```python
from build123d import *

# Parameters (mm, degrees)
BOSS_EXTRUDE1_DEPTH  = 6.35
SKETCH2_R            = 17
CUT_EXTRUDE1_DEPTH   = 109.352768769
M5_CLEARANCE_HOLE1_D = 5.5
M5_CLEARANCE_HOLE2_D = 5.5
FILLET1_R            = 5.08


with BuildPart() as part:
    # Sketch1 → Boss-Extrude1 (new body)
    with BuildSketch(Plane(origin=(0, 0, 0), x_dir=(1, 0, 0), z_dir=(0, 1, 0))):
        with BuildLine():
            Line((0, 60), (0, 0))
            Line((0, 0), (60, 0))
            Line((60, 0), (60, 60))
            ThreePointArc((60, 60), (30, 90), (0, 60))
        make_face()
    extrude(amount=BOSS_EXTRUDE1_DEPTH)

    # Sketch2 → Cut-Extrude1 (cut, through all)
    with BuildSketch(Plane(origin=(0, 6.35, 0), x_dir=(1, 0, 0), z_dir=(0, 1, 0))):
        with Locations(Location((30, 60, 0), (0, 0, 270))):
            Circle(SKETCH2_R)
    extrude(amount=-CUT_EXTRUDE1_DEPTH, mode=Mode.SUBTRACT)

    # M5 Clearance Hole1 (through all)
    with Locations(Plane(origin=(0, 6.35, 0), x_dir=(-1, 0, 0), z_dir=(0, 1, 0))):
        with Locations((-15.857864376, -74.142135624), (-44.142135624, -45.857864376), (-44.142135624, -74.142135624), (-15.857864376, -45.857864376), (-30, -80), (-50, -60), (-30, -40), (-10, -60)):
            Hole(M5_CLEARANCE_HOLE1_D / 2)

    # M5 Clearance Hole2 (through all)
    with Locations(Plane(origin=(0, 6.35, 0), x_dir=(-1, 0, 0), z_dir=(0, 1, 0))):
        with Locations((-10.95, -12.7), (-49.05, -12.7)):
            Hole(M5_CLEARANCE_HOLE2_D / 2)

    # Fillet1
    fillet1_edges = [part.edges().sort_by_distance(p)[0] for p in [
        (60, 3.175, 0),
        (0, 3.175, 0),
    ]]
    fillet(fillet1_edges, radius=FILLET1_R)


solid = part.part
```
Geometry: final body of the model. Coordinates: model frame, mm. Round coordinates to 2 decimals unless told otherwise and drop trailing zeros. Order: outer loops, then holes, each group sorted by start corner. A loop starts at its lowest first (then second) coordinate and runs counter-clockwise, first axis right, second up. Notation, with made-up numbers: (34, 79.5) - (72, 79.5) arc R26 ccw to (72, 108.5) - close; hole circle Ø11 at (-11, 12). An arc over 180 degrees is marked (long way). Write item = value, one per line. Start each with the question number.
Q1. Cut plane B-B on z = -12.7. Return the cut outline in (x, y), and give its area (3 significant figures).
Q2. Cut plane D-D on z = -44. Return the cut outline in (x, y).
Q3. Cut plane A-A on x = 30. Return the cut outline in (y, z), and give its area (3 significant figures).
Q4. Ray query, line 1 (X direction, y = 5.25, z = -12.5); line 2 (Z direction, x = 31.5, y = 4); line 3 (Z direction, x = 49.05, y = 3.75). Return the intervals inside material, ascending. Write a range as from..to.
Q5. Cut plane C-C on x = 49.05. Return the cut outline in (y, z).
Q6. Pull-direction query (X, two-part tool) for faces 1 (the cylindrical face through (30.66, 3.131, -89.993)), 2 (the flat face through (60, 3, -32)), 3 (the cylindrical face through (15, 3, -52)); classes: +X half, -X half, draft (parallel to the pull), parting line (faces both ways), or undercut.
Outcome:
q1.outline = (0, 0) - (8.2, 0) - (8.2, 6.35) - (0, 6.35) - close; (13.7, 0) - (46.3, 0) - (46.3, 6.35) - (13.7, 6.35) - close; (51.8, 0) - (60, 0) - (60, 6.35) - (51.8, 6.35) - close
q1.area = 311 mm^2
q2.outline = (0, 0) - (13.83, 0) - (13.83, 6.35) - (0, 6.35) - close; (17.89, 0) - (24.26, 0) - (24.26, 6.35) - (17.89, 6.35) - close; (35.74, 0) - (42.11, 0) - (42.11, 6.35) - (35.74, 6.35) - close; (46.17, 0) - (60, 0) - (60, 6.35) - (46.17, 6.35) - close
q3.outline = (0, -90) - (6.35, -90) - (6.35, -82.75) - (0, -82.75) - close; (0, -77.25) - (6.35, -77.25) - (6.35, -77) - (0, -77) - close; (0, -43) - (6.35, -43) - (6.35, -42.75) - (0, -42.75) - close; (0, -37.25) - (6.35, -37.25) - (6.35, 0) - (0, 0) - close
q3.area = 286 mm^2
q4.line_1 = 0..8.21, 13.69..46.31, 51.79..60
q4.line_2 = -89.96..-82.3, -77.7..-76.93, -43.07..-42.3, -37.7..0
q4.line_3 = -83.18..-62.58, -57.42..-15.45, -9.95..0
q5.outline = (0, -83.18) - (6.35, -83.18) - (6.35, -62.58) - (0, -62.58) - close; (0, -57.42) - (6.35, -57.42) - (6.35, -15.45) - (0, -15.45) - close; (0, -9.95) - (6.35, -9.95) - (6.35, 0) - (0, 0) - close
q6.face_1 = parting line
q6.face_2 = +X half
q6.face_3 = undercut
